Source: CAD feature listing. Evaluate the final solid. Frame: model axes, mm. A direction names the side the tool comes from. Give positions to 0.01 mm unless a question says otherwise; leave off trailing zeros. Loops run counter-clockwise (first coordinate to the right, second up) from the corner with the lowest first, then second, coordinate; pieces in that order, holes last.
```python
from build123d import *

# Parameters (mm, degrees)
F1_DEPTH = 152.4
F2_W     = 19.05
F2_H     = 152.4
F3_DEPTH = 19.05


with BuildPart() as f1:
    # F0 (on Front) → F1 (new body, symmetric)
    with BuildSketch(Plane.XZ):
        Polygon((239.3357296876, 273.8439301559), (378.5296995641, 134.6499602793), (378.5296995641, 161.5907286425), (252.8061138692, 287.3143143375), align=None)
    extrude(amount=F1_DEPTH, both=True)

    # F2 (on face) → F3 (cut)
    with BuildSketch(Plane(origin=(270.0602141033, 0, 270.0602141033), x_dir=(0.7071067812, 0, -0.7071067812), z_dir=(0.7071067812, 0, 0.7071067812))):
        with Locations((74.0240174423, -76.2)):
            Rectangle(F2_W, F2_H)
    extrude(amount=-F3_DEPTH, mode=Mode.SUBTRACT)


solid = f1.part
```
(1) First-contact query: pin 1 (8 mm diameter, centred on x = 327.5, y = 114.5, fed in from +Z); pin 2 (2 mm diameter, centred on x = 346.5, y = 18.5, fed in from -Z); pin 3 (6 mm diameter, centred on y = -15.5, z = 175, fed in from -X). Flat tips, straight axial feed; report the tip coordinate or a pass-through.
A:
pin 1: stops at z = 216.62
pin 2: stops at z = 165.68
pin 3: stops at x = 335.18
(2) Section B-B, the plane z = 200.5. Return the cut outline in (x, y), then the cut area to 3 significant figures.
A:
outline: (312.68, 0) - (318.66, 0) - (318.66, -152.4) - (339.62, -152.4) - (339.62, 152.4) - (312.68, 152.4) - close
area: 7,300 mm2
(3) Section D-D, the plane x = 367.5. Return the cut outline in (y, z), then the cut area to 3 significant figures.
A:
outline: (-152.4, 145.68) - (152.4, 145.68) - (152.4, 172.62) - (-152.4, 172.62) - close
area: 8,210 mm2
(4) Ray query, line 1 along Y through (x, z) = (319.5, 211); line 2 along X through (y, z) = (111, 235.5); line 3 along Z through (x, y) = (295, 0). Return the intervals inside material, ascending.
A:
line 1: y = 0 to 152.4
line 2: x = 277.68 to 304.62
line 3: z = 218.18 to 245.12
(5) Section A-A, the plane y = -68. Return the cut outline in (x, z).
A:
outline: (239.34, 273.84) - (302.2, 210.98) - (315.67, 224.45) - (252.81, 287.31) - close; (315.67, 197.51) - (378.53, 134.65) - (378.53, 161.59) - (329.14, 210.98) - close
(6) Section C-C, the plane y = 128. Return the cut outline in (x, z).
A:
outline: (239.34, 273.84) - (378.53, 134.65) - (378.53, 161.59) - (252.81, 287.31) - close
(7) Reachability of faces 1 (the flat face through (280, -152.4, 249)), 2 (the flat face through (316, 0, 211)) from +Z, -Z, +X, -X, +Y, -Y: full face, straight path, thin tool, end or side. Return the list, or none.
A:
face 1: +Z, -Z, +X, -X, -Y
face 2: -Y
